Input: part model. Units: mm. Frame: model coordinates. A direction names the side the tool comes from. Coordinates: 2 decimals unless noted, no trailing zeros. Order: outer loops, then holes, each group sorted by start corner. A loop starts at its lowest first (then second) coordinate and runs counter-clockwise, first axis right, second up.
from build123d import *

# Parameters (mm, degrees)
SKETCH_1_W             = 29
SKETCH_1_H             = 29
EXTRUDE_1_DEPTH        = 29
SKETCH_3_W             = 22.7
SKETCH_3_H             = 9
EXTRUDE_3_DEPTH        = 1
SKETCH_4_R             = 1
SKETCH_4_W             = 14
SKETCH_4_H             = 3
SKETCH_4_W_2           = 13
SKETCH_4_H_2           = 2
EXTRUDE_4_DEPTH        = 1
SKETCH_5_R             = 7.25
EXTRUDE_5_DEPTH        = 2.5
SKETCH_6_R             = 6
EXTRUDE_6_DEPTH        = 1
SKETCH_7_R             = 5
EXTRUDE_7_DEPTH        = 5.3
SKETCH_8_R             = 14
SKETCH_8_R_2           = 13
EXTRUDE_8_DEPTH        = 15
HOLE_WIZARD_M3_1_D     = 2.5
HOLE_WIZARD_M3_1_DEPTH = 4.2
HOLE_WIZARD_M3_1_TIP   = 0.751075774
FILLET_1_R             = 0.5


with BuildPart() as part:
    # 草图1 → 凸台-拉伸1 (new body)
    with BuildSketch(Plane(origin=(0, 0, 0), x_dir=(0, 0, -1), z_dir=(1, 0, 0))):
        Rectangle(SKETCH_1_W, SKETCH_1_H)
    extrude(amount=EXTRUDE_1_DEPTH)

    # 草图3 → 凸台-拉伸3 (add)
    with BuildSketch(Plane.ZY):
        with Locations((0, -8.6)):
            Rectangle(SKETCH_3_W, SKETCH_3_H)
    extrude(amount=EXTRUDE_3_DEPTH)

    # 草图4 → 凸台-拉伸4 (add)
    # profile 1 of 3: a face of its own
    with BuildSketch(Plane.ZY.offset(1)):
        with Locations((-9, -8.6)):
            Circle(SKETCH_4_R)
    # profile 2 of 3: a face of its own
    with BuildSketch(Plane.ZY.offset(1)):
        with Locations((9, -8.6)):
            Circle(SKETCH_4_R)
    # profile 3 of 3: a face of its own
    with BuildSketch(Plane.ZY.offset(1)):
        with Locations((0, -8.6)):
            Rectangle(SKETCH_4_W, SKETCH_4_H)
        with Locations((0, -8.6)):
            Rectangle(SKETCH_4_W_2, SKETCH_4_H_2, mode=Mode.SUBTRACT)
    extrude(amount=EXTRUDE_4_DEPTH)

    # 草图5 → 凸台-拉伸5 (add)
    with BuildSketch(Plane.ZY):
        with Locations((7.25, 7.25)):
            Circle(SKETCH_5_R)
    extrude(amount=EXTRUDE_5_DEPTH)

    # 草图6 → 凸台-拉伸6 (add)
    with BuildSketch(Plane.ZY.offset(2.5)):
        with Locations((7.25, 7.25)):
            Circle(SKETCH_6_R)
    extrude(amount=EXTRUDE_6_DEPTH)

    # 草图7 → 凸台-拉伸7 (add)
    with BuildSketch(Plane.ZY.offset(3.5)):
        with Locations((7.25, 7.25)):
            Circle(SKETCH_7_R)
    extrude(amount=EXTRUDE_7_DEPTH)

    # 草图8 → 凸台-拉伸8 (add)
    with BuildSketch(Plane(origin=(29, 0, 0), x_dir=(0, 0, -1), z_dir=(1, 0, 0))):
        with Locations(Location((0, 0, 0), (0, 0, 180))):
            Circle(SKETCH_8_R)
        Circle(SKETCH_8_R_2, mode=Mode.SUBTRACT)
    extrude(amount=EXTRUDE_8_DEPTH)

    # M3 螺纹孔1
    with Locations(Plane(origin=(0, -14.5, 0), x_dir=(-1, 0, 0), z_dir=(0, -1, 0))):
        with Locations((-26.7, 10), (-26.7, -10), (-3, 0)):
            Hole(HOLE_WIZARD_M3_1_D / 2, depth=HOLE_WIZARD_M3_1_DEPTH)
            with Locations((0, 0, -(HOLE_WIZARD_M3_1_DEPTH + HOLE_WIZARD_M3_1_TIP / 2))):  # 118° drill point
                Cone(0, HOLE_WIZARD_M3_1_D / 2, HOLE_WIZARD_M3_1_TIP, mode=Mode.SUBTRACT)

    # 圆角1
    fillet_1_edges = [part.edges().sort_by_distance(p)[0] for p in [
        (29, 0, 14.5),
        (29, -14.5, 0),
        (29, 0, -14.5),
        (29, 14.5, 0),
        (14.5, -14.5, -14.5),
        (14.5, -14.5, 14.5),
        (14.5, 14.5, 14.5),
        (14.5, 14.5, -14.5),
    ]]
    fillet(fillet_1_edges, radius=FILLET_1_R - 0.0001)  # a hair under: the kernel refuses the full size


solid = part.part
Item 1: Cut plane D-D on y = -1.75. Return loops of the section in (x, z), then the cut area to 3 significant figures.
Response values:
outline: (0, -14.5) - (28.5, -14.5) arc R0.5 ccw to (29, -14) - (29, -13.89) - (44, -13.89) - (44, -12.88) - (29, -12.88) - (29, 12.88) - (44, 12.88) - (44, 13.89) - (29, 13.89) - (29, 14) arc R0.5 ccw to (28.5, 14.5) - (0, 14.5) - close
area: 871 mm2
Item 2: Cut plane A-A on y = 9. Return loops of the section in (x, z), then the cut area to 3 significant figures.
Response values:
outline: (-8.8, 2.57) - (-3.5, 2.57) - (-3.5, 1.51) - (-2.5, 1.51) - (-2.5, 0.21) - (0, 0.21) - (0, -14.5) - (28.5, -14.5) arc R0.5 ccw to (29, -14) - (29, -10.72) - (44, -10.72) - (44, -9.38) - (29, -9.38) - (29, 9.38) - (44, 9.38) - (44, 10.72) - (29, 10.72) - (29, 14) arc R0.5 ccw to (28.5, 14.5) - (0, 14.5) - (0, 14.29) - (-2.5, 14.29) - (-2.5, 12.99) - (-3.5, 12.99) - (-3.5, 11.93) - (-8.8, 11.93) - close
area: 977 mm2
Item 3: Cut plane B-B on x = 39. Return loops of the section in (y, z).
Response values:
outline: circle Ø28 at (0, 0); hole circle Ø26 at (0, 0)
Item 4: Pin query (flat end, axial travel): pin 1 Ø0.8 at (x, y) = (-1.5, -8.5) entering from -Z; pin 2 Ø0.5 at (x, z) = (-1.5, -1) entering from +Y; pin 3 Ø0.5 at (x, z) = (-1.5, 2) entering from +Y; pin 4 Ø6 at (y, z) = (9.5, 12) entering from -X. Return the tip coordinate at first contact, or that it passes through.
Response values:
pin 1: stops at z = -10
pin 2: stops at y = -7.1
pin 3: stops at y = 12.5
pin 4: stops at x = -8.8
Item 5: Access query for faces 1 (the face through (-2.99, 11.31, 2.83)), 2 (the face through (27.89, -12.37, 9.62)), 3 (the face through (0, 13, 13)). Directions: +Z, -Z, +X, -X, +Y, -Y. A direction counts if a zero-diameter tool reaches every point of the face in a straight line with its end or side. Return the directions, or none.
Response values:
face 1: -X
face 2: -Y
face 3: +Z, -X, +Y
Item 6: Draft query along Z for faces 4 (the face through (-1.493, -9.576, 8.783)), 5 (the face through (-6.11, 8.75, 12.02)), 6 (the face through (14, 0, 14.5)). Return one class per face: pulls with the +Z half, pulls with the -Z half, needs draft (parallel to the pull), parting line crosses it, or undercut.
Response values:
face 4: undercut
face 5: parting line crosses it
face 6: pulls with the +Z half
Item 7: Ray query, probe 1 along Z at (x, y) = (26.7, -12); probe 2 along Y at (x, z) = (34.75, 0); probe 3 along X at (y, z) = (-13.35, 10). Return the intervals inside material, ascending.
Response values:
probe 1: z = -14.5 to -11.25, -8.75 to 8.75, 11.25 to 14.5
probe 2: y = -14 to -13, 13 to 14
probe 3: x = 0 to 25.45, 27.95 to 29
Item 8: Cut plane C-C on y = -5.25. Return loops of the section in (x, z), then the cut area to 3 significant figures.
Response values:
outline: (-1, -11.35) - (0, -11.35) - (0, -14.5) - (28.5, -14.5) arc R0.5 ccw to (29, -14) - (29, -12.98) - (44, -12.98) - (44, -11.89) - (29, -11.89) - (29, 11.89) - (44, 11.89) - (44, 12.98) - (29, 12.98) - (29, 14) arc R0.5 ccw to (28.5, 14.5) - (0, 14.5) - (0, 11.35) - (-1, 11.35) - close
area: 896 mm2
